Read the model definition and answer for the solid it produces. Units are mm, in the model's axes. A direction names the side the tool comes from. Coordinates: 2 decimals unless noted, no trailing zeros. Order: outer loops, then holes, each group sorted by start corner. A loop starts at its lowest first (then second) coordinate and runs counter-clockwise, first axis right, second up. Notation, with made-up numbers: (25, 12) - (73, 12) arc R25 ccw to (73, 24) - close; hole circle Ø10 at (-6, 58). An arc over 180 degrees is marked (long way). Answer as a JSON object with one key per item and string values. Group by question number.
from build123d import *

# Parameters (mm, degrees)
SKETCH2_W           = 19.66
SKETCH2_H           = 8.2
BOSS_EXTRUDE1_DEPTH = 2
SKETCH3_R           = 2.6
BOSS_EXTRUDE2_DEPTH = 7
FILLET1_R           = 1


with BuildPart() as part:
    # Sketch2 → Boss-Extrude1 (new body)
    with BuildSketch(Plane(origin=(0, 0, 0), x_dir=(1, 0, 0), z_dir=(0, 1, 0))):
        Rectangle(SKETCH2_W, SKETCH2_H)
    extrude(amount=BOSS_EXTRUDE1_DEPTH)

    # Sketch3 → Boss-Extrude2 (add)
    with BuildSketch(Plane(origin=(0, 2, 0), x_dir=(1, 0, 0), z_dir=(0, 1, 0))):
        with Locations((-5.73, 0)):
            Circle(SKETCH3_R)
        with Locations((5.73, 0)):
            Circle(SKETCH3_R)
    extrude(amount=BOSS_EXTRUDE2_DEPTH)

    # Fillet1
    fillet1_edges = [part.edges().sort_by_distance(p)[0] for p in [
        (-8.33, 9, 0),
        (3.13, 9, 0),
    ]]
    fillet(fillet1_edges, radius=FILLET1_R)


solid = part.part
1. A cutting plane is placed at C-C on z = 0. Write down the section's boundary in (x, y).
2. A cutting plane is placed at B-B on y = 7. Write down the section's boundary in (x, z).
3. For a pull along X with two mould halves and no side action, classify faces 3 (the flat face through (-9.83, 1, 0)), 4 (the flat face through (0, 1, -4.1)), 5 (the cylindrical face through (-3.25, 4.96, -0.78)), 6 (the flat face through (0, 2, 0)) as pulls with the +X half, pulls with the -X half, needs draft (parallel to the pull), parting line crosses it, or undercut.
4. A cutting plane is placed at A-A on x = -5.73. Write down the section's boundary in (y, z), and give its area (3 significant figures).
5. For faces 1 (the flat face through (9.83, 1, 0)), 2 (the cylindrical face through (8.21, 4.96, -0.78)), determine the directions among +Z, -Z, +X, -X, +Y, -Y from which every point of the face is accessible in a straight line to the end or side of a thin tool.
6. Given pin 1 (4 mm diameter, centred on x = -3, y = 7.5, fed in from -Z), flat-ended and moving along its own axis, determine where the tip first touches the part or whether it passes through.
7. A cutting plane is placed at D-D on z = 3.75. Write down the section's boundary in (x, y), and give its area (3 significant figures).
8. Straight lines are drawn through the part: L1, parallel to Y at x = 3, z = -0.75; L2, parallel to X at y = 7.5, z = -1; L3, parallel to X at y = 3, z = 1.5. For each, find the intervals that lie inside material, in ascending order.
Derived:
{
 "1": {"outline": "(-9.83, 0) - (9.83, 0) - (9.83, 2) - (8.33, 2) - (8.33, 8) arc R1 ccw to (7.33, 9) - (4.13, 9) arc R1 ccw to (3.13, 8) - (3.13, 2) - (-3.13, 2) - (-3.13, 8) arc R1 ccw to (-4.13, 9) - (-7.33, 9) arc R1 ccw to (-8.33, 8) - (-8.33, 2) - (-9.83, 2) - close"},
 "2": {"outline": "circle Ø5.2 at (-5.73, 0); circle Ø5.2 at (5.73, 0)"},
 "3": {"face 3": "pulls with the -X half", "face 4": "needs draft", "face 5": "undercut", "face 6": "undercut"},
 "4": {"outline": "(0, -4.1) - (2, -4.1) - (2, -2.6) - (8, -2.6) arc R1 ccw to (9, -1.6) - (9, 1.6) arc R1 ccw to (8, 2.6) - (2, 2.6) - (2, 4.1) - (0, 4.1) - close", "area": "52.4 mm2"},
 "5": {"face 1": "+Z, -Z, +X, +Y, -Y", "face 2": "+Y"},
 "6": {"pin 1": "stops at z = -2.5"},
 "7": {"outline": "(-9.83, 0) - (9.83, 0) - (9.83, 2) - (-9.83, 2) - close", "area": "39.3 mm2"},
 "8": {"L1": "y = 0 to 2", "L2": "x = -8.13 to -3.33, 3.33 to 8.13", "L3": "x = -7.85 to -3.61, 3.61 to 7.85"}
}
